Read the model definition and answer for the solid it produces. Units are mm, in the model's axes. A direction names the side the tool comes from. Coordinates: 2 decimals unless noted, no trailing zeros. Order: outer loops, then holes, each group sorted by start corner. A loop starts at its lowest first (then second) coordinate and runs counter-clockwise, first axis right, second up. Notation, with made-up numbers: M 3,67.5 L 61,67.5 A14 ccw 61,93.5 Z; hole C 3,13 d7. An arc over 180 degrees is marked long. Use a Markdown table: item, result. Add a question column.
1) For faces 4 (the face through (0, 12, -68)), 5 (the face through (2.535, 13.132, -12.475)), determine the directions among +Z, -Z, +X, -X, +Y, -Y from which every point of the face is accessible in a straight line to the end or side of a thin tool.
2) The mould has two halves that part along Y. Classify faces 1 (the face through (-44.048, 12.066, -142.465)), 2 (the face through (2, 25, -94)), 3 (the face through (-0.9, 12.32, -139.14)): released by +Y, released by -Y, zero draft, split by the parting line, or undercut.
3) Find section B-B on x = -46. Write down the section's boundary in (y, z), plus the area to 3 significant figures.
4) Find section A-A on y = 12.5. Write down the section's boundary in (x, z).
5) Each of these flat-tipped pins is pushed along its axis until it touches: pin 1 Ø4 at (y, z) = (12.5, -14) entering from -X; pin 2 Ø8 at (x, y) = (-8.5, 11.5) entering from +Z. Where does it stop, or does it pass through?
6) Find section C-C on z = -14. Write down the section's boundary in (x, y), plus the area to 3 significant figures.
7) Find the intervals of material crossed by probe 1 along Z at (x, y) = (3.5, 12.5); probe 2 along X at (y, z) = (19.5, -118); probe 3 along Z at (x, y) = (-52, 15), in increasing order. Write a range as [from, to].
8) Find section D-D on x = -35. Write down the section's boundary in (y, z), plus the area to 3 significant figures.
Autodesk Inventor part; units mm, degrees
ref_plane "YZ Plane" through (0, 0, 0) normal (1, 0, 0) x (0, 1, 0)
ref_plane "XZ Plane" through (0, 0, 0) normal (0, 1, 0) x (-1, 0, 0)
ref_plane "XY Plane" through (0, 0, 0) normal (0, 0, 1) x (1, 0, 0)
sketch "Sketch1" plane through (0, 0, 0) normal (0, 1, 0) x (-1, 0, 0)
  line L0 (0, 0) -> (0, -137)
  line L1 (3, -140) -> (56, -140)
  arc A0 (0, -137) -> (3, -140) centre (3, -137) ccw
  line L2 (56, -145) -> (3, -145)
  arc A1 (-5, -137) -> (3, -145) centre (3, -137) ccw
  line L3 (-5, -137) -> (-5, 0)
  line L4 (56, -140) -> (56, -145)
  line L5 (-5, 0) -> (0, 0)
  point P0 (0, -140)
  dimension "d0" = 140
  dimension "d1" = 56
  dimension "d2" = 3
  dimension "d3" = 5
extrude "Extrusion1" add sketch "Sketch1" along normal blind 25
sketch "Sketch2" plane through (-3, 0, -145) normal (0, 0, -1) x (-1, 0, 0)
  line L0 (53, 0) -> (0, 0)
  line L1 (53, 0) -> (53, 25)
  line L2 (0, 25) -> (53, 25)
  line L3 (0, 0) -> (0, 25)
  circle A0 centre (43, 12.5) radius 2
  point P0 (-3, 0)
  dimension "d6" = 4
  dimension "d7" = 12.5
  dimension "d8" = 10
hole "Hole1" at (-46, 12.5, -145) direction (0, 0, 1) diameter 4 end through all
sketch "Sketch3" plane through (0, 0, -137) normal (-1, 0, 0) x (0, 0, 1)
  line L0 (137, 0) -> (0, 0)
  line L1 (137, 0) -> (137, 25)
  line L2 (0, 25) -> (137, 25)
  line L3 (0, 0) -> (0, 25)
  circle A0 centre (123, 12.5) radius 2
  circle A1 centre (133, 12.5) radius 2
  dimension "d16" = 4
  dimension "d17" = 4
  dimension "d18" = 4
  dimension "d19" = 14
  dimension "d20" = 12.5
  dimension "d21" = 12.5
hole "Hole2" at (0, 12.5, -14) at (0, 12.5, -4) direction (1, 0, 0) diameter 3.302 end through all
properties part number "Brazo"
Check result:
| question | item | result |
|---|---|---|
| 1 | face 4 | +Z, -X, +Y, -Y |
| 1 | face 5 | +X, -X |
| 2 | face 1 | undercut |
| 2 | face 2 | released by +Y |
| 2 | face 3 | zero draft |
| 3 | outline | M 0,-145 L 10.5,-145 L 10.5,-140 L 0,-140 Z; M 14.5,-145 L 25,-145 L 25,-140 L 14.5,-140 Z |
| 3 | area | 105 mm2 |
| 4 | outline | M -56,-145 L -48,-145 L -48,-140 L -56,-140 Z; M -44,-145 L -3,-145 A8 ccw 5,-137 L 5,-15.65 L 0,-15.65 L 0,-137 A3 cw -3,-140 L -44,-140 Z; M 0,-12.35 L 5,-12.35 L 5,-5.65 L 0,-5.65 Z; M 0,-2.35 L 5,-2.35 L 5,0 L 0,0 Z |
| 5 | pin 1 | stops at x = 0 |
| 5 | pin 2 | stops at z = -140 |
| 6 | outline | M 0,0 L 5,0 L 5,10.85 L 0,10.85 Z; M 0,14.15 L 5,14.15 L 5,25 L 0,25 Z |
| 6 | area | 108 mm2 |
| 7 | probe 1 | z = [-141.66, -15.65], [-12.35, -5.65], [-2.35, 0] |
| 7 | probe 2 | x = [0, 5] |
| 7 | probe 3 | z = [-145, -140] |
| 8 | outline | M 0,-145 L 25,-145 L 25,-140 L 0,-140 Z |
| 8 | area | 125 mm2 |
